The model under review builds one solid part; all positions refer to its coordinate system, in mm. A direction names the side the tool comes from. Coordinates: 2 decimals unless noted, no trailing zeros. Write each loop counter-clockwise with the first axis right and the second up, starting at its lowest first coordinate (ties: lowest second). Pieces come first, ordered by that corner, then holes. Notation, with made-up numbers: M 72.25,51 L 90.25,51 A20 ccw 90.25,75 Z; hole C 45,57 d11. An arc over 180 degrees is marked long. Answer as a JSON object with one key per item and string values.
```python
from build123d import *

# Parameters (mm, degrees)
SKETCH1_R           = 5
SKETCH1_R_2         = 2.5
BOSS_EXTRUDE1_DEPTH = 4
SKETCH2_R           = 4.275
SKETCH2_R_2         = 3.2
CUT_EXTRUDE1_DEPTH  = 0.1
SKETCH3_R           = 4.275
SKETCH3_R_2         = 3.2
CUT_EXTRUDE2_DEPTH  = 0.1


with BuildPart() as part:
    # Sketch1 → Boss-Extrude1 (new body)
    with BuildSketch(Plane(origin=(0, 0, 0), x_dir=(1, 0, 0), z_dir=(0, 1, 0))):
        Circle(SKETCH1_R)
        Circle(SKETCH1_R_2, mode=Mode.SUBTRACT)
    extrude(amount=BOSS_EXTRUDE1_DEPTH)

    # Sketch2 → Cut-Extrude1 (cut)
    with BuildSketch(Plane(origin=(0, 4, 0), x_dir=(1, 0, 0), z_dir=(0, 1, 0))):
        Circle(SKETCH2_R)
        Circle(SKETCH2_R_2, mode=Mode.SUBTRACT)
    extrude(amount=-CUT_EXTRUDE1_DEPTH, mode=Mode.SUBTRACT)

    # Sketch3 → Cut-Extrude2 (cut)
    with BuildSketch(Plane.XZ):
        Circle(SKETCH3_R)
        Circle(SKETCH3_R_2, mode=Mode.SUBTRACT)
    extrude(amount=-CUT_EXTRUDE2_DEPTH, mode=Mode.SUBTRACT)


solid = part.part
```
(1) For faces 1 (the face through (2, 0.1, -3)), 2 (the face through (-0.54, 1.97, 2.44)), list the 3-axis set-ups (+Z, -Z, +X, -X, +Y, -Y) from which the entire face can be reached by the end or side of a thin tool; tool diameter is ignored.
Results list:
{"face 1": "-Y", "face 2": "+Y, -Y"}
(2) Add section A-A on x = 0. Give the boundary of the cut face in (y, z) (3 decimals).
Results list:
{"outline": "M 0,-5 L 4,-5 L 4,-4.275 L 3.9,-4.275 L 3.9,-3.2 L 4,-3.2 L 4,-2.5 L 0,-2.5 L 0,-3.2 L 0.1,-3.2 L 0.1,-4.275 L 0,-4.275 Z; M 0,2.5 L 4,2.5 L 4,3.2 L 3.9,3.2 L 3.9,4.275 L 4,4.275 L 4,5 L 0,5 L 0,4.275 L 0.1,4.275 L 0.1,3.2 L 0,3.2 Z"}
(3) Draft analysis for pull direction Z (two halves, no side actions). For faces 3 (the face through (-1.08, 1.97, 4.88)), 4 (the face through (4, 0, -2)), 5 (the face through (2, 3.9, 3)), state which applies: released by +Z, released by -Z, zero draft, split by the parting line, or undercut.
Results list:
{"face 3": "split by the parting line", "face 4": "zero draft", "face 5": "undercut"}
(4) Add section B-B on z = 1. Give the boundary of the cut face in (x, y), and give its area (3 significant figures).
Results list:
{"outline": "M -4.9,0 L -4.16,0 L -4.16,0.1 L -3.04,0.1 L -3.04,0 L -2.29,0 L -2.29,4 L -3.04,4 L -3.04,3.9 L -4.16,3.9 L -4.16,4 L -4.9,4 Z; M 2.29,0 L 3.04,0 L 3.04,0.1 L 4.16,0.1 L 4.16,0 L 4.9,0 L 4.9,4 L 4.16,4 L 4.16,3.9 L 3.04,3.9 L 3.04,4 L 2.29,4 Z", "area": "20.4 mm²"}
(5) Add section C-C on y = 0.85. Give the boundary of the cut face in (x, z).
Results list:
{"outline": "C 0,0 d10; hole C 0,0 d5"}
(6) For pin 1 Ø1.5 at (y, z) = (2.5, 3) entering from -X; pin 2 Ø1 at (y, z) = (1.5, 3.5) entering from +X, all flat-tipped, find the tip position at first contact; note any pin that passes through.
Results list:
{"pin 1": "x = -4.47", "pin 2": "x = 4"}
(7) Wall thickness on line 1 along Z through (x, y) = (0, 0.05) (3 decimals); line 2 along X through (y, z) = (1.2, 0): over which ranges is each line inside the solid? List them lowest first. Write a range as from..to.
Results list:
{"line 1": "-5..-4.275, -3.2..-2.5, 2.5..3.2, 4.275..5", "line 2": "-5..-2.5, 2.5..5"}
(8) Add section D-D on z = -4. Give the boundary of the cut face in (x, y), and give its area (3 significant figures).
Results list:
{"outline": "M -3,0 L -1.51,0 L -1.51,0.1 L 1.51,0.1 L 1.51,0 L 3,0 L 3,4 L 1.51,4 L 1.51,3.9 L -1.51,3.9 L -1.51,4 L -3,4 Z", "area": "23.4 mm²"}
